CAD build for the part. Positions are in the model's coordinates, mm. Coordinates: 2 decimals unless noted, no trailing zeros. Loops run counter-clockwise (first coordinate to the right, second up) from the corner with the lowest first, then second, coordinate; pieces in that order, holes last. Notation, with made-up numbers: (-34.75, 39.5) -> (18.25, 39.5) arc R27 ccw to (18.25, 57.5) -> close; hole circle Ø9 at (-23.75, 26.25). An arc over 180 degrees is marked (long way). Write each question's results on one line, items separated by ' | '.
from build123d import *

# Parameters (mm, degrees)
SKETCH1_R           = 9.525
SKETCH1_R_2         = 7.874
BOSS_EXTRUDE1_DEPTH = 152.4
BOSS_EXTRUDE2_START = -3.175
SKETCH2_R           = 9.525
BOSS_EXTRUDE2_DEPTH = 3.175
SKETCH3_R           = 2.778125
CUT_EXTRUDE1_DEPTH  = 12.7
CIRPATTERN1_COUNT   = 2
CIRPATTERN1_ANGLE   = 90
SKETCH4_R           = 2.778125
CUT_EXTRUDE2_DEPTH  = 12.7
CIRPATTERN2_COUNT   = 2
CIRPATTERN2_ANGLE   = 90


with BuildPart() as part:
    # Sketch1 → Boss-Extrude1 (new body)
    with BuildSketch(Plane(origin=(0, 0, 0), x_dir=(0, 0, -1), z_dir=(1, 0, 0))):
        with Locations(Location((0, 0, 0), (0, 0, 180))):
            Circle(SKETCH1_R)
        with Locations(Location((0, 0, 0), (0, 0, 180))):
            Circle(SKETCH1_R_2, mode=Mode.SUBTRACT)
    extrude(amount=BOSS_EXTRUDE1_DEPTH)

    # Sketch2 → Boss-Extrude2 (add)
    with BuildSketch(Plane(origin=(0, 0, 0), x_dir=(0, 0, -1), z_dir=(1, 0, 0)).offset(BOSS_EXTRUDE2_START)):
        with Locations(Location((0, 0, 0), (0, 0, 180))):
            Circle(SKETCH2_R)
    extrude(amount=BOSS_EXTRUDE2_DEPTH)

    # Sketch3 → Cut-Extrude1 (cut, symmetric)
    with BuildSketch(Plane.XY):
        with Locations((6.35, 0)):
            Circle(SKETCH3_R)
    cut_extrude1 = extrude(amount=CUT_EXTRUDE1_DEPTH, both=True, mode=Mode.SUBTRACT)

    # CirPattern1: Cut-Extrude1 ×2 about axis
    cirpattern1_axis = Axis((152.4, 0, 0), (-1, 0, 0))
    for i in range(1, CIRPATTERN1_COUNT):
        add(cut_extrude1.rotate(cirpattern1_axis, i * CIRPATTERN1_ANGLE / (CIRPATTERN1_COUNT - 1)), mode=Mode.SUBTRACT)

    # Sketch4 → Cut-Extrude2 (cut, symmetric)
    with BuildSketch(Plane(origin=(0, 0, 0), x_dir=(1, 0, 0), z_dir=(0, -0.7071067811865488, 0.7071067811865464))):
        with Locations(Location((12.7, 0, 0), (0, 0, 270))):
            Circle(SKETCH4_R)
    cut_extrude2 = extrude(amount=CUT_EXTRUDE2_DEPTH, both=True, mode=Mode.SUBTRACT)

    # CirPattern2: Cut-Extrude2 ×2 about axis
    cirpattern2_axis = Axis((152.4, 0, 0), (-1, 0, 0))
    for i in range(1, CIRPATTERN2_COUNT):
        add(cut_extrude2.rotate(cirpattern2_axis, i * CIRPATTERN2_ANGLE / (CIRPATTERN2_COUNT - 1)), mode=Mode.SUBTRACT)


solid = part.part
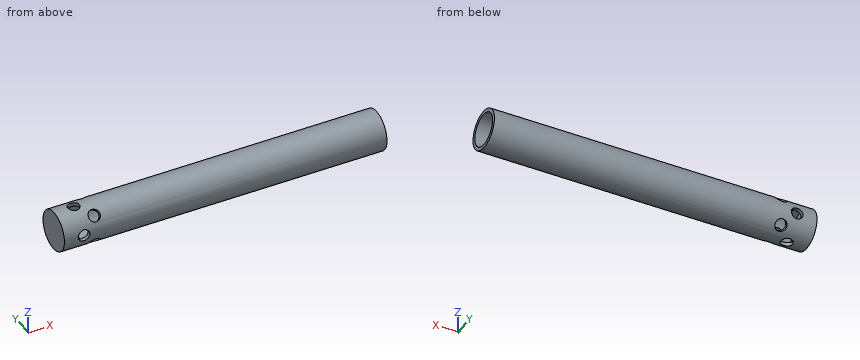
1) Slice it at A-A (y = 0). Write the cut outline in (x, z) (3 decimals), then the cut area to 3 significant figures.
Outcome:
outline: (-3.175, -9.525) -> (3.572, -9.525) -> (3.572, -7.874) -> (0, -7.874) -> (0, 7.874) -> (3.572, 7.874) -> (3.572, 9.525) -> (-3.175, 9.525) -> close; (9.128, -9.525) -> (152.4, -9.525) -> (152.4, -7.874) -> (9.128, -7.874) -> close; (9.128, 7.874) -> (152.4, 7.874) -> (152.4, 9.525) -> (9.128, 9.525) -> close | area: 545 mm^2
2) Slice it at C-C (x = 6.35). Write the cut outline in (y, z) (3 decimals), then the cut area to 3 significant figures.
Outcome:
outline: (-9.111, -2.778) arc R9.525 ccw to (-2.778, -9.111) -> (-2.778, -7.368) arc R7.874 cw to (-7.368, -2.778) -> close; (-9.111, 2.778) -> (-7.368, 2.778) arc R7.874 cw to (-2.778, 7.368) -> (-2.778, 9.111) arc R9.525 ccw to start; (2.778, -9.111) arc R9.525 ccw to (9.111, -2.778) -> (7.368, -2.778) arc R7.874 cw to (2.778, -7.368) -> close; (2.778, 7.368) arc R7.874 cw to (7.368, 2.778) -> (9.111, 2.778) arc R9.525 ccw to (2.778, 9.111) -> close | area: 52.9 mm^2
3) Drill centre lines: L1, parallel to Y at x = 35.5, z = 0 (3 decimals); L2, parallel to X at y = 5.25, z = 0 (3 decimals); L3, parallel to X at y = -8.65, z = 0 (3 decimals). Where is each one in solid material? Low to high. Write a range as from..to.
Outcome:
L1: y = -9.525..-7.874, 7.874..9.525 | L2: x = -3.175..0 | L3: x = -3.175..3.572, 9.128..152.4
4) Pin check, flat tips, straight feed: pin 1 (4.5 mm diameter, centred on y = 0.5, z = -0.5, fed in from +X); pin 2 (5 mm diameter, centred on x = 27, z = 4, fed in from -Y); pin 3 (3 mm diameter, centred on x = 76, z = -3.5, fed in from -Y). Stop position of each tip, or through.
Outcome:
pin 1: stops at x = 0 | pin 2: stops at y = -9.41 | pin 3: stops at y = -9.31
5) Slice it at D-D (x = 123). Write the cut outline in (y, z) (3 decimals), then the cut area to 3 significant figures.
Outcome:
outline: circle Ø19.05 at (0, 0); hole circle Ø15.748 at (0, 0) | area: 90.2 mm^2
